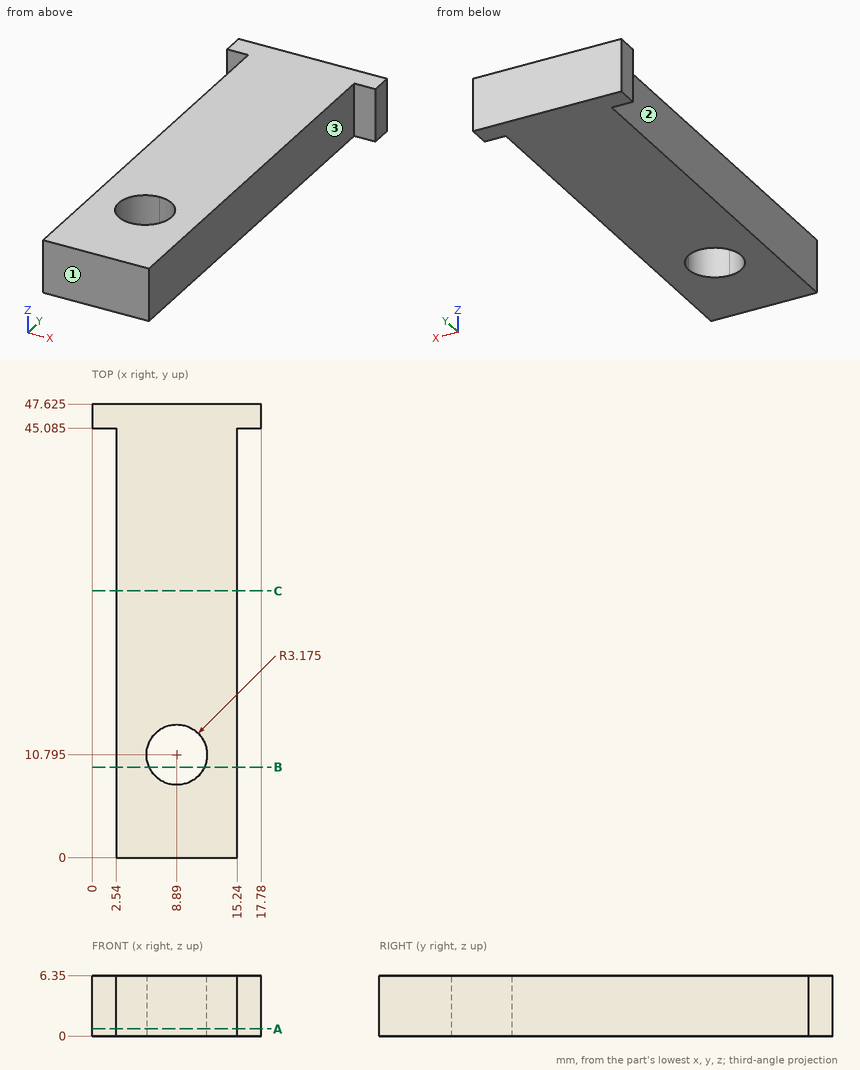
Check sheet for the drawn part. Datum: minimum x, y, z corner. Units: mm. A direction names the side the tool comes from. Give positions to 0.01 mm unless a question says otherwise; leave off trailing zeros. Write each loop counter-clockwise with the first axis right and the second up, starting at its lowest first coordinate (ties: lowest second). Pieces come first, ordered by that corner, then holes.
(1) Cross-section at A-A (z = 0.75). Enter the section's corners in (x, y) (3 decimals).
(2) Cross-section at B-B (y = 9.5). Enter the section's corners in (x, z), plus the area to 3 significant figures.
(3) Access from +Z, -Z, +X, -X, +Y, -Y to the whole of each face (thin tool, end or side, straight path). Record for the marked faces 1, 2 and 3.
(4) Cross-section at C-C (y = 28). Enter the section's corners in (x, z).
(5) Material ranges on line 1 (X direction, y = 18.5, z = 4.5); line 2 (Y direction, x = 16, z = 3) (3 decimals); line 3 (Y direction, x = 10.25, z = 2) (3 decimals), recorded low to high.
(6) Gauge pin test, flat ends, axial feed: pin 1 (1.9 mm diameter, centred on y = 26, z = 4.5, fed in from -X); pin 2 (3 mm diameter, centred on x = 1, z = 2.5, fed in from -Y) (3 decimals); pin 3 (1.9 mm diameter, centred on y = 29, z = 3, fed in from +X). Record the tip position at first contact, or that the pin passes through.
Worked out:
1. outline: (0, 45.085) - (2.54, 45.085) - (2.54, 0) - (15.24, 0) - (15.24, 45.085) - (17.78, 45.085) - (17.78, 47.625) - (0, 47.625) - close; hole circle Ø6.35 at (8.89, 10.795)
2. outline: (2.54, 0) - (5.99, 0) - (5.99, 6.35) - (2.54, 6.35) - close; (11.79, 0) - (15.24, 0) - (15.24, 6.35) - (11.79, 6.35) - close
2. area: 43.8 mm2
3. face 1: +Z, -Z, +X, -X, -Y
3. face 2: +Z, -Z, -X, -Y
3. face 3: +Z, -Z, +X, -Y
4. outline: (2.54, 0) - (15.24, 0) - (15.24, 6.35) - (2.54, 6.35) - close
5. line 1: x = 2.54 to 15.24
5. line 2: y = 45.085 to 47.625
5. line 3: y = 0 to 7.926, 13.664 to 47.625
6. pin 1: stops at x = 2.54
6. pin 2: stops at y = 45.085
6. pin 3: stops at x = 15.24
